```python
from build123d import *

# Parameters (mm, degrees)
SKETCH_1_R      = 1.5
EXTRUDE_1_DEPTH = 5


with BuildPart() as part:
    # Эскиз1 → Бобышка-Вытянуть1 (new body)
    with BuildSketch(Plane(origin=(0, 0, 0), x_dir=(1, 0, 0), z_dir=(0, 1, 0))):
        with BuildLine():
            Line((0, 10), (0, 2.5))
            ThreePointArc((0, 2.5), (0.956708581, 2.309698831), (1.767766953, 1.767766953))
            Line((1.767766953, 1.767766953), (3.556747109, 3.556747109))
            ThreePointArc((3.556747109, 3.556747109), (3.556747109, 5.678067453), (5.678067453, 5.678067453))
            Line((5.678067453, 5.678067453), (7.071067812, 7.071067812))
            ThreePointArc((7.071067812, 7.071067812), (3.826834324, 9.238795325), (0, 10))
        make_face()
        with BuildLine():
            ThreePointArc((2.5, 0), (-1.767766953, -1.767766953), (0, 2.5))
            Line((0, 2.5), (0, 10))
            ThreePointArc((0, 10), (-7.071067812, -7.071067812), (10, 0))
            ThreePointArc((10, 0), (9.238795325, 3.826834324), (7.071067812, 7.071067812))
            Line((7.071067812, 7.071067812), (5.678067453, 5.678067453))
            ThreePointArc((5.678067453, 5.678067453), (6.00322658, 5.19143243), (6.117407281, 4.617407281))
            ThreePointArc((6.117407281, 4.617407281), (5.19143243, 3.231587982), (3.556747109, 3.556747109))
            Line((3.556747109, 3.556747109), (1.767766953, 1.767766953))
            ThreePointArc((1.767766953, 1.767766953), (2.309698831, 0.956708581), (2.5, 0))
        make_face()
        with Locations((-4.617407281, -4.617407281)):
            Circle(SKETCH_1_R, mode=Mode.SUBTRACT)
        with Locations((4.617407281, -4.617407281)):
            Circle(SKETCH_1_R, mode=Mode.SUBTRACT)
        with Locations((-4.617407281, 4.617407281)):
            Circle(SKETCH_1_R, mode=Mode.SUBTRACT)
    extrude(amount=EXTRUDE_1_DEPTH)


solid = part.part
```
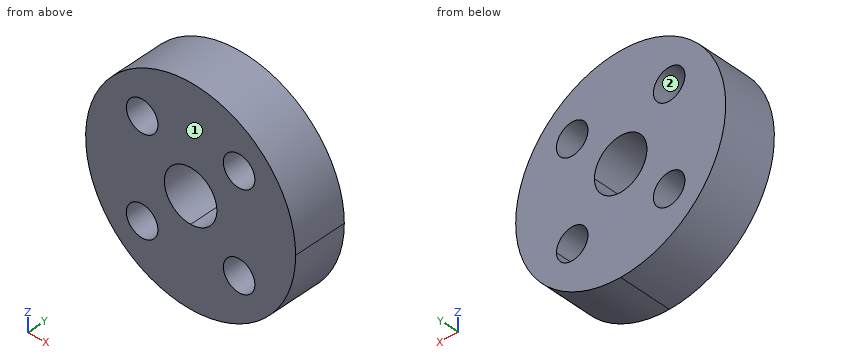
Geometry: final body of the model. Coordinates: model frame, mm. Face numbers are marked on the shaded views. Coordinates: 2 decimals unless noted, no trailing zeros. Order: outer loops, then holes, each group sorted by start corner. A loop starts at its lowest first (then second) coordinate and runs counter-clockwise, first axis right, second up. Notation, with made-up numbers: (70.25, -10.75) - (78.25, -10.75) arc R28 ccw to (78.25, 18.25) - close; hole circle Ø3 at (-18, -37). An arc over 180 degrees is marked (long way). Write each question's results on one line, items separated by ' | '.
1) Pull-direction query (Z, two-part tool) for the marked faces 1 and 2; classes: pulls with the +Z half, pulls with the -Z half, needs draft (parallel to the pull), parting line crosses it, or undercut.
Results list:
face 1: needs draft | face 2: undercut
2) Section B-B, the plane z = -1.5. Return loops of the section in (x, y).
Results list:
outline: (-9.89, 0) - (-2, 0) - (-2, 5) - (-9.89, 5) - close; (2, 0) - (9.89, 0) - (9.89, 5) - (2, 5) - close
3) Section C-C, the plane y = 1.65. Return loops of the section in (x, z), plus the area to 3 significant figures.
Results list:
outline: circle Ø20 at (0, 0); hole circle Ø3 at (-4.62, -4.62); hole circle Ø3 at (-4.62, 4.62); hole circle Ø5 at (0, 0); hole circle Ø3 at (4.62, -4.62); hole circle Ø3 at (4.62, 4.62) | area: 266 mm^2
4) Pin query (flat end, axial travel): pin 1 (1.5 mm diameter, centred on y = 2, z = -4, fed in from +X); pin 2 (2 mm diameter, centred on x = 5, y = 1, fed in from +Z). Return the tip coordinate at first contact, or that it passes through.
Results list:
pin 1: x = 9.46 | pin 2: z = 9.17
5) Section A-A, the plane x = -2.25. Return loops of the section in (y, z).
Results list:
outline: (0, -9.74) - (5, -9.74) - (5, -1.09) - (0, -1.09) - close; (0, 1.09) - (5, 1.09) - (5, 9.74) - (0, 9.74) - close
6) Line query: line 1 (Z direction, x = 0, y = 3.9); line 2 (X direction, y = 3.65, z = 5.25). Output: solid intervals per line, ascending. Write a range as from..to.
Results list:
line 1: -10..-2.5, 2.5..10 | line 2: -8.51..-5.98, -3.26..3.26, 5.98..8.51
7) Section D-D, the plane x = -5.5. Return loops of the section in (y, z).
Results list:
outline: (0, -8.35) - (5, -8.35) - (5, -5.83) - (0, -5.83) - close; (0, -3.4) - (5, -3.4) - (5, 3.4) - (0, 3.4) - close; (0, 5.83) - (5, 5.83) - (5, 8.35) - (0, 8.35) - close
